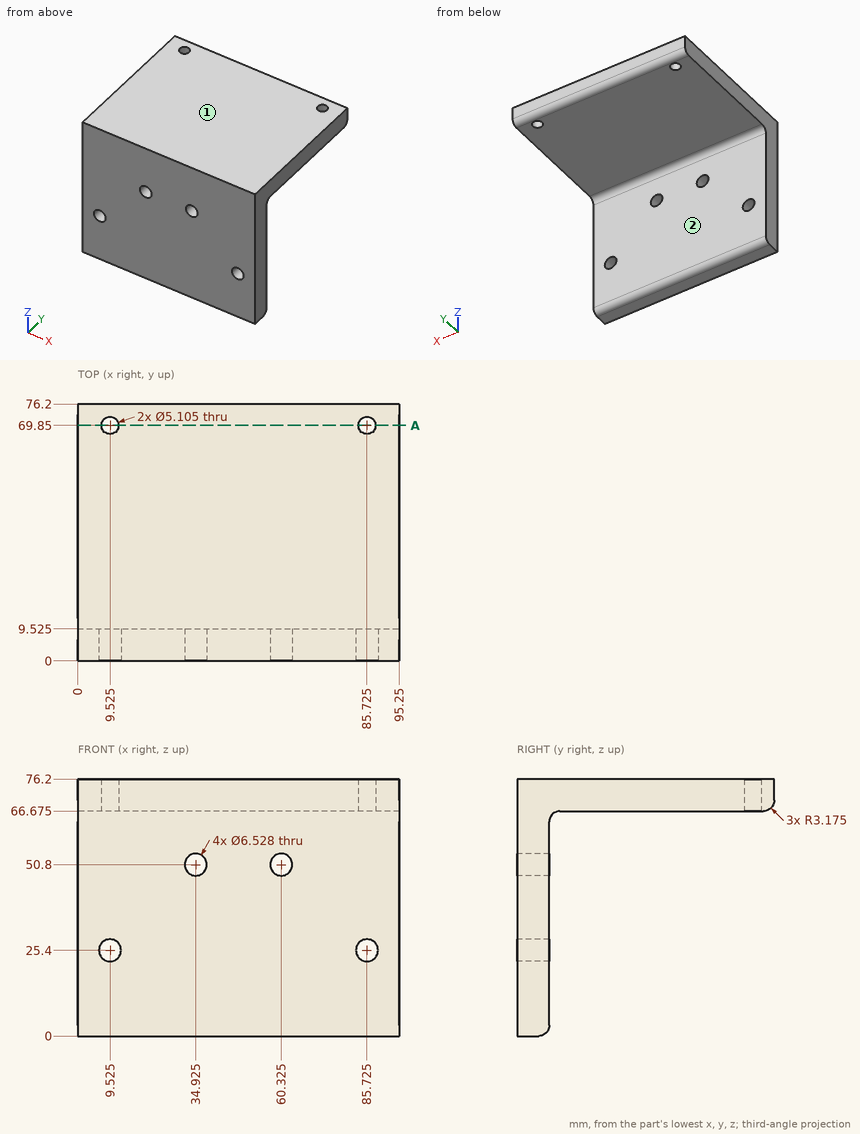
Can you work these out from the drawing? Everything is in mm from the part's minimum corner. A direction names the side the tool comes from. Give positions to 0.01 mm unless a question says otherwise; leave off trailing zeros.
1. Will this pin go through, and if not, where does the flat tip stop? P1, Ø8, axis at x = 85, z = 57.5, coming from the -Y side.
2. For the marked faces 1 and 2, which set-ups out of +Z, -Z, +X, -X, +Y, -Y let a thin tool reach every point of the face, with its end or its side?
3. Suppose I cut it at A-A (y = 69.85). Give the number of separate pieces and of enclosed holes in the cut face, plus the area to 3 significant figures.
4. I need wall thicknesses on L1, parallel to X at y = 3, z = 50; L2, parallel to Z at x = 18, y = 26.5 (1 decimal); L3, parallel to Y at x = 90.5, z = 36 (1 decimal). Which ranges of each line are inside material? Lowest first, please.
Solved:
1. P1: stops at y = 0
2. face 1: +Z, +X, -X, +Y, -Y
2. face 2: -Z, +X, -X, +Y
3. separate pieces: 3
3. enclosed holes: 0
3. area: 810 mm2
4. L1: x = 0 to 31.76, 38.09 to 57.16, 63.49 to 95.25
4. L2: z = 66.7 to 76.2
4. L3: y = 0 to 9.5
